Geometry: final body of the model. Coordinates: model frame, mm. A direction names the side the tool comes from. Round coordinates to 2 decimals unless told otherwise and drop trailing zeros. Loops run counter-clockwise (first coordinate to the right, second up) from the corner with the lowest first, then second, coordinate; pieces in that order, holes last. Notation, with made-up numbers: M 45,86 L 74,86 A13 ccw 74,93 Z; hole C 62.25,71.5 d10. An arc over 180 degrees is marked long. Answer as a JSON object with one key per item and string values.
from build123d import *

# Parameters (mm, degrees)
F0_W     = 27.051
F0_H     = 5.08
F1_DEPTH = 6.35
F2_DEPTH = 1.016
F3_R     = 1.0795
F4_DEPTH = 6.351
F3_R_2   = 2.413
F5_DEPTH = 1.016
F6_R     = 2.54
F7_R     = 0.508


with BuildPart() as f1:
    # F0 (on Top) → F1 (new body)
    with BuildSketch(Plane.XY):
        with BuildLine():
            Line((5.1615120301, 0), (0, 0))
            Line((0, 0), (0, -25.4))
            Line((0, -25.4), (3.175, -38.1))
            Line((3.175, -38.1), (34.925, -38.1))
            Line((34.925, -38.1), (38.1, -25.4))
            Line((38.1, -25.4), (38.1, 0))
            Line((38.1, 0), (32.9384879699, 0))
            ThreePointArc((32.9384879699, 0), (34.184496322, -3.4072309325), (34.6075, -7.0104))
            ThreePointArc((34.6075, -7.0104), (15.4468309325, -22.144896322), (5.1615120301, 0))
        make_face()
        with Locations((19.05, -31.75)):
            Rectangle(F0_W, F0_H, mode=Mode.SUBTRACT)
        with BuildLine():
            Line((32.9384879699, 0), (5.1615120301, 0))
            ThreePointArc((5.1615120301, 0), (15.4468309325, -22.144896322), (34.6075, -7.0104))
            ThreePointArc((34.6075, -7.0104), (34.184496322, -3.4072309325), (32.9384879699, 0))
        make_face()
    extrude(amount=F1_DEPTH)

    # F0 (on Top) → F2 (cut)
    with BuildSketch(Plane.XY):
        with BuildLine():
            Line((32.9384879699, 0), (5.1615120301, 0))
            ThreePointArc((5.1615120301, 0), (15.4468309325, -22.144896322), (34.6075, -7.0104))
            ThreePointArc((34.6075, -7.0104), (34.184496322, -3.4072309325), (32.9384879699, 0))
        make_face()
    extrude(amount=F2_DEPTH, mode=Mode.SUBTRACT)

    # F3 (on face) → F4 (cut, through all)
    with BuildSketch(Plane.XY.offset(6.35)):
        with Locations((6.35, -23.277434341)):
            Circle(F3_R)
        with Locations((31.75, -23.277434341)):
            Circle(F3_R)
    extrude(amount=-F4_DEPTH, mode=Mode.SUBTRACT)

    # F3 (on face) → F5 (cut)
    with BuildSketch(Plane.XY.offset(6.35)):
        with Locations((31.75, -23.277434341)):
            Circle(F3_R_2)
        with Locations((31.75, -23.277434341)):
            Circle(F3_R, mode=Mode.SUBTRACT)
        with Locations((6.35, -23.277434341)):
            Circle(F3_R_2)
        with Locations((6.35, -23.277434341)):
            Circle(F3_R, mode=Mode.SUBTRACT)
    extrude(amount=-F5_DEPTH, mode=Mode.SUBTRACT)

    # F6
    f6_edges = [f1.edges().sort_by_distance(p)[0] for p in [
        (38.1, -12.7, 6.35),
        (36.5125, -31.75, 6.35),
        (19.05, -38.1, 6.35),
        (1.5875, -31.75, 6.35),
        (0, -12.7, 6.35),
        (19.05, 0, 6.35),
    ]]
    fillet(f6_edges, radius=F6_R)

    # F7
    f7_edges = [f1.edges().sort_by_distance(p)[0] for p in [
        (5.5245, -31.75, 6.35),
        (19.05, -34.29, 6.35),
        (19.05, -29.21, 6.35),
        (32.5755, -31.75, 6.35),
    ]]
    fillet(f7_edges, radius=F7_R)


solid = f1.part
1) Section query B-B (x = 6.35). Return the cut outline in (y, z).
Results:
{"outline": "M -38.1,0 L -34.29,0 L -34.29,5.84 A0.51 ccw -34.8,6.35 L -35.56,6.35 A2.54 ccw -38.1,3.81 Z; M -29.21,0 L -24.36,0 L -24.36,5.33 L -25.69,5.33 L -25.69,6.35 L -28.7,6.35 A0.51 ccw -29.21,5.84 Z; M -22.2,0 L -16,0 L -16,1.02 L 0,1.02 L 0,3.81 A2.54 ccw -2.54,6.35 L -20.86,6.35 L -20.86,5.33 L -22.2,5.33 Z"}
2) Ray query, line 1 (Y direction, x = 6.35, z = 3.85); line 2 (Y direction, x = 21, z = 1.5); line 3 (Z direction, x = 28.5, y = -4). Return the intervals inside material, ascending.
Results:
{"line 1": "-38.1 to -34.29, -29.21 to -24.36, -22.2 to 0", "line 2": "-38.1 to -34.29, -29.21 to 0", "line 3": "1.02 to 6.35"}
3) Pin query (flat end, axial travel): P1, Ø1.5, axis at y = -29, z = 4, coming from the -X side; P2, Ø11.5, axis at x = 26.5, y = -6, coming from the -Z side; P3, Ø2, axis at y = -25, z = 5.5, coming from the -X side. Return the tip coordinate at first contact, or that it passes through.
Results:
{"P1": "x = 0.72", "P2": "z = 1.02", "P3": "x = 0.1"}
4) Section query A-A (x = 19.05). Return the cut outline in (y, z), and give its area (3 significant figures).
Results:
{"outline": "M -38.1,0 L -34.29,0 L -34.29,5.84 A0.51 ccw -34.8,6.35 L -35.56,6.35 A2.54 ccw -38.1,3.81 Z; M -29.21,0 L -22.57,0 L -22.57,1.02 L 0,1.02 L 0,3.81 A2.54 ccw -2.54,6.35 L -28.7,6.35 A0.51 ccw -29.21,5.84 Z", "area": "184 mm2"}
5) Section query C-C (y = -19). Return the cut outline in (x, z), and give its area (3 significant figures).
Results:
{"outline": "M 0,0 L 9.14,0 L 9.14,1.02 L 28.96,1.02 L 28.96,0 L 38.1,0 L 38.1,3.81 A2.54 ccw 35.56,6.35 L 2.54,6.35 A2.54 ccw 0,3.81 Z", "area": "219 mm2"}
6) Pull-direction query (X, two-part tool) for faces 4 (the flat face through (36.5, -31.8, 1.9)), 5 (the cylindrical face through (34.05, -22.55, 5.85)), 6 (the cylindrical face through (8.65, -22.55, 5.85)), 7 (the flat face through (1.565, -31.661, 1.878)); classes: +X half, -X half, draft (parallel to the pull), parting line (faces both ways), or undercut.
Results:
{"face 4": "+X half", "face 5": "undercut", "face 6": "undercut", "face 7": "-X half"}
7) Reachability of faces 1 (the flat face through (38.1, -13, 2)), 2 (the flat face through (19, -29.21, 3)), 3 (the flat face through (6, -22, 5.334)) from +Z, -Z, +X, -X, +Y, -Y: full face, straight path, thin tool, end or side. Return the list, or none.
Results:
{"face 1": "+Z, -Z, +X, +Y, -Y", "face 2": "+Z, -Z", "face 3": "+Z"}
8) Section query D-D (x = 23). Return the cut outline in (y, z), and give its area (3 significant figures).
Results:
{"outline": "M -38.1,0 L -34.29,0 L -34.29,5.84 A0.51 ccw -34.8,6.35 L -35.56,6.35 A2.54 ccw -38.1,3.81 Z; M -29.21,0 L -22.06,0 L -22.06,1.02 L 0,1.02 L 0,3.81 A2.54 ccw -2.54,6.35 L -28.7,6.35 A0.51 ccw -29.21,5.84 Z", "area": "184 mm2"}
